```python
from build123d import *

# Parameters (mm, degrees)
SKETCH1_R           = 11
SKETCH1_R_2         = 10
BOSS_EXTRUDE1_DEPTH = 486.5
SKETCH3_R           = 3.25
CUT_EXTRUDE1_DEPTH  = 488.166931009


with BuildPart() as part:
    # Sketch1 → Boss-Extrude1 (new body)
    with BuildSketch(Plane.XY):
        Circle(SKETCH1_R)
        Circle(SKETCH1_R_2, mode=Mode.SUBTRACT)
    extrude(amount=-BOSS_EXTRUDE1_DEPTH)

    # Sketch3 → Cut-Extrude1 (cut, through all)
    with BuildSketch(Plane(origin=(10.767604694, 2.249152987, 0), x_dir=(0, 0, -1), z_dir=(0.978873153981486, 0.20446845334754707, 0))):
        with Locations(Location((32, 0, 0), (0, 0, 90))):
            Circle(SKETCH3_R)
        with Locations(Location((170.5, 0, 0), (0, 0, 90))):
            Circle(SKETCH3_R)
        with Locations(Location((454.5, 0, 0), (0, 0, 90))):
            Circle(SKETCH3_R)
    extrude(amount=-CUT_EXTRUDE1_DEPTH, mode=Mode.SUBTRACT)


solid = part.part
```
Geometry: final body of the model. Coordinates: model frame, mm. Round coordinates to 2 decimals unless told otherwise and drop trailing zeros. Loops run counter-clockwise (first coordinate to the right, second up) from the corner with the lowest first, then second, coordinate; pieces in that order, holes last.
Item 1: Line query: L1, parallel to Y at x = 0, z = -281.5; L2, parallel to Z at x = 9.75, y = 4; L3, parallel to X at y = -1, z = -209. Output: solid intervals per line, ascending.
Checked values:
L1: y = -11 to -10, 10 to 11
L2: z = -486.5 to -457.12, -451.88 to -173.12, -167.88 to -34.62, -29.38 to 0
L3: x = -10.95 to -9.95, 9.95 to 10.95
Item 2: Mould query, pull axis X, two halves, no side actions, for faces 1 (the flat face through (2, -10, -486.5)), 2 (the cylindrical face through (-2.17, -9.76, -239.84)), 3 (the cylindrical face through (-2.38, -10.74, -239.84)). Classes: released by +X, released by -X, zero draft, split by the parting line, or undercut.
Checked values:
face 1: zero draft
face 2: undercut
face 3: split by the parting line
Item 3: Section B-B, the plane z = -408. Output: boundary loops of the cut face in (x, y).
Checked values:
outline: circle Ø22 at (0, 0); hole circle Ø20 at (0, 0)
Item 4: Contact query for flat-ended pins moving along their axis: P1, Ø1, axis at x = 5, z = -64, coming from the -Y side; P2, Ø2, axis at y = 8, z = -78.5, coming from the -X side; P3, Ø2, axis at x = -1.5, z = -201, coming from the +Y side; P4, Ø10, axis at x = -4, z = -431, coming from the -Y side. Output: stop coordinate, or through.
Checked values:
P1: stops at y = -10.04
P2: stops at x = -8.49
P3: stops at y = 10.99
P4: stops at y = -11
Item 5: Section A-A, the plane x = 0. Output: boundary loops of the cut face in (y, z).
Checked values:
outline: (-11, -486.5) - (-10, -486.5) - (-10, 0) - (-11, 0) - close; (10, -486.5) - (11, -486.5) - (11, 0) - (10, 0) - close
